```python
from build123d import *

# Parameters (mm, degrees)
F0_W     = 40
F0_H     = 40
F0_W_2   = 9.4724982
F0_H_2   = 96
F0_W_3   = 9.4725108908
F1_DEPTH = 3


# Not quite as in the source:
# - ends of sketch curves that miss each other by under 0.0002 mm in the source are joined


with BuildPart() as f1:
    # F0 (on Front) → F1 (new body)
    with BuildSketch(Plane.XZ):
        with BuildLine():
            ThreePointArc((86.0931563339, 18.3499035886), (87.5338209496, 28.3038164709), (88.0155156934, 38.3499035886))
            ThreePointArc((88.0155156934, 38.3499035886), (60.5384552721, 109.1679368787), (-7.5119860033, 142.9217534139))
            Line((-7.5119860033, 142.9217534139), (-7.5119861066, 46.9217522737))
            Line((-7.5119861066, 46.9217522737), (-16.9844843066, 46.9217522737))
            Line((-16.9844843066, 46.9217522737), (-16.9844843066, 38.3499035886))
            Line((-16.9844843066, 38.3499035886), (-16.9844843066, 18.3499035886))
            Line((-16.9844843066, 18.3499035886), (7.9387861441, 18.3499035886))
            Line((7.9387861441, 18.3499035886), (-12.4932068051, 26.3993963716))
            Line((-12.4932068051, 26.3993963716), (-8.6108822672, 35.0509963625))
            Line((-8.6108822672, 35.0509963625), (-5.9856059721, 42.9176116083))
            Line((-5.9856059721, 42.9176116083), (56.3745017477, 18.3499035886))
            Line((56.3745017477, 18.3499035886), (86.0931563339, 18.3499035886))
        make_face()
        with Locations((38.3114193761, 61.7765981326)):
            Rectangle(F0_W, F0_H, mode=Mode.SUBTRACT)
        with Locations((-12.2482352066, 94.9217522737)):
            Rectangle(F0_W_2, F0_H_2)
        with BuildLine():
            ThreePointArc((69.1839553915, -21.6500964114), (79.7291121051, -2.533837301), (86.0931563339, 18.3499035886))
            Line((86.0931563339, 18.3499035886), (56.3745017477, 18.3499035886))
            Line((56.3745017477, 18.3499035886), (83.3328157811, 7.7292678634))
            Line((83.3328157811, 7.7292678634), (80.2973141438, 0.0242670983))
            Line((80.2973141438, 0.0242670983), (76.8252149481, -8.7889473734))
            Line((76.8252149481, -8.7889473734), (7.9387861441, 18.3499035886))
            Line((7.9387861441, 18.3499035886), (-16.9844843066, 18.3499035886))
            Line((-16.9844843066, 18.3499035886), (69.1839553915, -21.6500964114))
        make_face()
        with Locations((-21.720739752, 94.9217522737)):
            Rectangle(F0_W_3, F0_H_2)
        with BuildLine():
            ThreePointArc((47.3344412398, -44.6445288546), (59.1325161296, -33.9771469845), (69.1839553915, -21.6500964114))
            Line((69.1839553915, -21.6500964114), (-16.9844843066, 18.3499035886))
            Line((-16.9844843066, 18.3499035886), (-103.1529240046, -21.6500964114))
            ThreePointArc((-103.1529240046, -21.6500964114), (-93.1014847427, -33.9771469845), (-81.3034098529, -44.6445288546))
            Line((-81.3034098529, -44.6445288546), (-56.1818756669, -44.6445288546))
            Line((-56.1818756669, -44.6445288546), (-16.9844843066, -21.6500964114))
            Line((-16.9844843066, -21.6500964114), (22.2130476509, -44.6445288546))
            Line((22.2130476509, -44.6445288546), (47.3344412398, -44.6445288546))
        make_face()
        Polygon((83.3328157811, 7.7292678634), (56.3745017477, 18.3499035886), (7.9387861441, 18.3499035886), (76.8252149481, -8.7889473734), (80.2973141438, 0.0242670983), align=None)
        Polygon((7.9387861441, 18.3499035886), (56.3745017477, 18.3499035886), (-5.9856059721, 42.9176116083), (-8.6108822672, 35.0509963625), (-12.4932068051, 26.3993963716), align=None)
        with BuildLine():
            Line((-26.4569951974, 46.9217522737), (-26.4569951974, 142.9217522737))
            ThreePointArc((-26.4569951974, 142.9217522737), (-100.9274442474, 101.4258853595), (-120.062124947, 18.3499035886))
            Line((-120.062124947, 18.3499035886), (-93.5930420098, 18.3499035886))
            Line((-93.5930420098, 18.3499035886), (-28.4441302912, 44.0163031416))
            Line((-28.4441302912, 44.0163031416), (-25.3580863459, 35.0509963625))
            Line((-25.3580863459, 35.0509963625), (-21.5126400611, 26.4221312691))
            Line((-21.5126400611, 26.4221312691), (-42.002340903, 18.3499035886))
            Line((-42.002340903, 18.3499035886), (-16.9844843066, 18.3499035886))
            Line((-16.9844843066, 18.3499035886), (-16.9844843066, 38.3499035886))
            Line((-16.9844843066, 38.3499035886), (-16.9844843066, 46.9217522737))
            Line((-16.9844843066, 46.9217522737), (-26.4569951974, 46.9217522737))
        make_face()
        with Locations((-72.2803842399, 61.7765981326)):
            Rectangle(F0_W, F0_H, mode=Mode.SUBTRACT)
        with BuildLine():
            Line((-103.1529240046, -21.6500964114), (-16.9844843066, 18.3499035886))
            Line((-16.9844843066, 18.3499035886), (-42.002340903, 18.3499035886))
            Line((-42.002340903, 18.3499035886), (-110.8216826256, -8.7625174025))
            ThreePointArc((-110.8216826256, -8.7625174025), (-107.2176813721, -15.3433934543), (-103.1529240046, -21.6500964114))
        make_face()
        with BuildLine():
            Line((-93.5930420098, 18.3499035886), (-120.062124947, 18.3499035886))
            ThreePointArc((-120.062124947, 18.3499035886), (-119.0172144252, 13.5643839342), (-117.750256284, 8.8328034975))
            Line((-117.750256284, 8.8328034975), (-93.5930420098, 18.3499035886))
        make_face()
        with BuildLine():
            Line((-110.8216826256, -8.7625174025), (-42.002340903, 18.3499035886))
            Line((-42.002340903, 18.3499035886), (-93.5930420098, 18.3499035886))
            Line((-93.5930420098, 18.3499035886), (-117.750256284, 8.8328034975))
            ThreePointArc((-117.750256284, 8.8328034975), (-117.7294799239, 8.7619692561), (-117.7086537702, 8.6911496387))
            Line((-117.7086537702, 8.6911496387), (-114.2904528488, 0.0147449249))
            Line((-114.2904528488, 0.0147449249), (-110.8722519274, -8.6616597888))
            ThreePointArc((-110.8722519274, -8.6616597888), (-110.8469808232, -8.7120953879), (-110.8216826256, -8.7625174025))
        make_face()
        Polygon((-93.5930420098, 18.3499035886), (-42.002340903, 18.3499035886), (-21.5126400611, 26.4221312691), (-25.3580863459, 35.0509963625), (-28.4441302912, 44.0163031416), align=None)
        with Locations((38.3114193761, 61.7765981326)):
            Rectangle(F0_W, F0_H)
        with Locations((-72.2803842399, 61.7765981326)):
            Rectangle(F0_W, F0_H)
    extrude(amount=F1_DEPTH)


solid = f1.part
```
Can you work these out from the model? Positions are in its coordinate system, mm. A direction names the side the tool comes from. Round coordinates to 2 decimals unless told otherwise and drop trailing zeros. Loops run counter-clockwise (first coordinate to the right, second up) from the corner with the lowest first, then second, coordinate; pieces in that order, holes last.
Item 1: Suppose I cut it at C-C, the plane z = 128. Write out the boundary of the cut face in (x, y).
Item 2: Which directions (+Z, -Z, +X, -X, +Y, -Y) give clear straight access to the entire face, cutting with the end or side of a thin tool? Please do faces 1 (the flat face through (-36.86, -1.48, -33.31)), 2 (the flat face through (-18, -3, 50)).
Item 3: Suppose I cut it at B-B, the plane x = 63.5. Write out the boundary of the cut face in (y, z), then the cut area to 3 significant figures.
Item 4: If we mould it in two halves opening along X, with no side actions, what happens to faces 3 (the flat face through (2.34, -1.479, -32.986)), 4 (the flat face through (-18, 0, 50))? For each: +X half, -X half, draft (parallel to the pull), parting line (faces both ways), or undercut.
Item 5: Please list where these lines run through material, in increasing order: L1, parallel to Z at x = -17, y = -2.7; L2, parallel to X at y = -2.75, z = -22; L3, parallel to X at y = -2.35, z = -20.5.
Reported:
1. outline: (-71.65, -3) - (37.68, -3) - (37.68, 0) - (-71.65, 0) - close
2. face 1: -Z, +Y, -Y
2. face 2: +Z, -Z, +X, -X, -Y
3. outline: (-3, -29.08) - (0, -29.08) - (0, 105.78) - (-3, 105.78) - close
3. area: 405 mm2
4. face 3: undercut
4. face 4: draft
5. L1: z = -21.66 to 142.92
5. L2: x = -102.91 to -17.58, -16.39 to 68.94
5. L3: x = -103.94 to 69.97
